from build123d import *

# Parameters (mm, degrees)
F3_D           = 6.6
F3_CBORE_D     = 11.25
F3_CBORE_DEPTH = 6
F5_DEPTH       = 52.071


with BuildPart() as f1:
    # F0 (on Right) → F1 (revolve)
    with BuildSketch(Plane.YZ):
        Polygon((-52.07, 0), (0, 0), (0, 27.94), (-44.069, 27.94), (-44.069, 39.6875), (-52.07, 39.6875), align=None)
    revolve(axis=Axis((0, -34.9322228922, 0), (0, 1, 0)))

    # F3 (through all)
    with Locations(Plane.XZ.offset(52.07)):
        with Locations((0, 33.3502), (-28.8821204213, -16.6751), (28.8821204213, -16.6751)):
            CounterBoreHole(F3_D / 2, F3_CBORE_D / 2, F3_CBORE_DEPTH)

    # F4 (on face) → F5 (cut, through all)
    with BuildSketch(Plane.XZ.offset(52.07)):
        with BuildLine():
            ThreePointArc((39.6875, 0), (34.0797569223, 20.3388255405), (18.8412474335, 34.9300021672))
            Line((18.8412474335, 34.9300021672), (39.6708929478, -1.1480021672))
            ThreePointArc((39.6708929478, -1.1480021672), (39.6833480198, -0.57406114), (39.6875, 0))
        make_face()
        with BuildLine():
            Line((-39.6708929478, -1.1480021672), (-18.8412474335, 34.9300021672))
            ThreePointArc((-18.8412474335, 34.9300021672), (-34.3703832127, 19.84375), (-39.6708929478, -1.1480021672))
        make_face()
        with BuildLine():
            ThreePointArc((-20.8296455143, -33.782), (0, -39.6875), (20.8296455143, -33.782))
            Line((20.8296455143, -33.782), (-20.8296455143, -33.782))
        make_face()
    extrude(amount=-F5_DEPTH, mode=Mode.SUBTRACT)


solid = f1.part
Model file for the job. Use its own axes, mm. A direction names the side the tool comes from. Give positions to 0.01 mm unless a question says otherwise; leave off trailing zeros. Order: outer loops, then holes, each group sorted by start corner. A loop starts at its lowest first (then second) coordinate and runs counter-clockwise, first axis right, second up. Notation, with made-up numbers: M 87,-16 L 91,-16 A11 cw 91,-11 Z; hole C -18.5,30.25 d8. An arc over 180 degrees is marked long. Write item = value, one per line.
Q1. Cut at B-B, the plane z = 24. List the corners of the cut face in (x, y).
Derived:
outline = M -25.15,-52.07 L 25.15,-52.07 L 25.15,-44.07 L 14.31,-44.07 L 14.31,0 L -14.31,0 L -14.31,-44.07 L -25.15,-44.07 Z
Q2. Cut at A-A, the plane x = 0. List the corners of the cut face in (y, z), then the cut area to 3 significant figures.
Derived:
outline = M -52.07,-33.78 L -44.07,-33.78 L -44.07,-27.94 L 0,-27.94 L 0,27.94 L -44.07,27.94 L -44.07,30.05 L -46.07,30.05 L -46.07,27.73 L -52.07,27.73 Z; M -52.07,38.98 L -46.07,38.98 L -46.07,36.65 L -44.07,36.65 L -44.07,39.69 L -52.07,39.69 Z
area = 2,970 mm2
Q3. Two-plate mould, pull along Z, no slides. Class faces 4 (the cylindrical face through (34.507, -48.126, -19.605)), 5 (the flat face through (0, 0, 0)), 6 (the cylindrical face through (24.42, -49.11, -20.1)), 7 (the flat face through (-26, -46.07, -19)): pulls with the +Z half, pulls with the -Z half, needs draft (parallel to the pull), parting line crosses it, or undercut.
Derived:
face_4 = pulls with the -Z half
face_5 = needs draft
face_6 = undercut
face_7 = undercut
Q4. Cut at D-D, the plane y = -10.5. List the corners of the cut face in (x, z).
Derived:
outline = C 0,0 d55.88
Q5. Flat gauge pins, fed straight in: pin 1 (3 mm diameter, centred on y = -6, z = -13, fed in from +X); pin 2 (5.5 mm diameter, centred on x = 28, z = -17.5, fed in from -Y); pin 3 (2 mm diameter, centred on y = -24.5, z = -17.5, fed in from -X). Where does each tip first touch, or does it go through?
Derived:
pin_1 = 25.46
pin_2 = -46.07
pin_3 = -22.55
Q6. Drill centre lines: line 1 (Z direction, x = 7.5, y = -47); line 2 (Z direction, x = 15.5, y = -11); line 3 (Z direction, x = -32, y = -49.5). Where is each one in solid material? Low to high. Write a range as [from, to].
Derived:
line_1 = [-33.78, 38.97]
line_2 = [-23.25, 23.25]
line_3 = [-23.48, -21.36], [-11.99, 12.14]
Q7. Cut at C-C, the plane x = -10.5. List the corners of the cut face in (y, z), then the cut area to 3 significant figures.
Derived:
outline = M -52.07,-33.78 L -44.07,-33.78 L -44.07,-25.89 L 0,-25.89 L 0,25.89 L -44.07,25.89 L -44.07,38.27 L -52.07,38.27 Z
area = 2,860 mm2
Q8. Tool access for faces 1 (the flat face through (28.8, -46.07, -20.3)), 2 (the cylindrical face through (27.7, -22.34, -3.64)), 3 (the cylindrical face through (-31.93, -45.06, -17.94)): list every direction of +Z, -Z, +X, -X, +Y, -Y with a clear straight run to the whole face (end or side of a thin tool).
Derived:
face_1 = -Y
face_2 = +Y
face_3 = +Y, -Y
